Read the model definition and answer for the solid it produces. Units are mm, in the model's axes. Face numbers are marked on the shaded views. Give positions to 0.01 mm unless a question says otherwise; leave off trailing zeros. Write each loop counter-clockwise with the first axis right and the second up, starting at its lowest first coordinate (ties: lowest second). Pieces come first, ordered by that corner, then holes. Notation, with made-up numbers: (81.25, 55) -> (87.25, 55) arc R26 cw to (87.25, 78) -> close; hole circle Ø7 at (-24.5, 42.25). An arc over 180 degrees is marked (long way). Use a Markdown table: item, result.
from build123d import *

# Parameters (mm, degrees)
SKETCH_1_W                          = 1077
SKETCH_1_H                          = 1947
SM_BASE_FLANGE_1_DEPTH              = 2
SM_EDGE_FLANGE_1_STRIP_W            = 9.5
SM_EDGE_FLANGE_1_STRIP_H            = 2
SM_EDGE_FLANGE_1_STRIP_CUT_DEPTH    = 1947
SM_EDGE_FLANGE_1_STRIP_2_W          = 9.5
SM_EDGE_FLANGE_1_STRIP_2_H          = 2
SM_EDGE_FLANGE_1_STRIP_CUT_2_DEPTH  = 1947
SM_EDGE_FLANGE_1_DEPTH              = 1947
SM_EDGE_FLANGE_1_BEND_DEPTH         = 1947
SM_EDGE_FLANGE_2_STRIP_W            = 9.5
SM_EDGE_FLANGE_2_STRIP_H            = 2
SM_EDGE_FLANGE_2_STRIP_CUT_DEPTH    = 1031.5
SM_EDGE_FLANGE_2_RELIEF_W           = 10.5
SM_EDGE_FLANGE_2_RELIEF_H           = 1
SM_EDGE_FLANGE_2_RELIEF_CUT_DEPTH   = 2
SM_EDGE_FLANGE_2_STRIP_2_W          = 9.5
SM_EDGE_FLANGE_2_STRIP_2_H          = 2
SM_EDGE_FLANGE_2_STRIP_CUT_2_DEPTH  = 1031.5
SM_EDGE_FLANGE_2_RELIEF_2_W         = 10.5
SM_EDGE_FLANGE_2_RELIEF_2_H         = 1
SM_EDGE_FLANGE_2_RELIEF_CUT_2_DEPTH = 2
SM_EDGE_FLANGE_2_DEPTH              = 1031.5
SM_EDGE_FLANGE_2_BEND_DEPTH         = 1031.5


# Sheet-metal steps are written as plain solids
with BuildPart() as part:
    # Sketch 1 → Базовая кромка1 (new body)
    with BuildSketch(Plane.XY):
        Rectangle(SKETCH_1_W, SKETCH_1_H)
    extrude(amount=SM_BASE_FLANGE_1_DEPTH)

    # Ребро-кромка1 strip (across the edge) → Ребро-кромка1 strip cut (cut)
    with BuildSketch(Plane(origin=(-538.5, -973.5, 0), x_dir=(1, 0, 0), z_dir=(0, 1, 0))):
        with Locations((-2, -1)):
            Rectangle(SM_EDGE_FLANGE_1_STRIP_W, SM_EDGE_FLANGE_1_STRIP_H)
    extrude(amount=SM_EDGE_FLANGE_1_STRIP_CUT_DEPTH, mode=Mode.SUBTRACT)

    # Ребро-кромка1 strip 2 (across the edge) → Ребро-кромка1 strip cut 2 (cut)
    with BuildSketch(Plane(origin=(538.5, 973.5, 0), x_dir=(-1, 0, 0), z_dir=(0, -1, 0))):
        with Locations((-2, -1)):
            Rectangle(SM_EDGE_FLANGE_1_STRIP_2_W, SM_EDGE_FLANGE_1_STRIP_2_H)
    extrude(amount=SM_EDGE_FLANGE_1_STRIP_CUT_2_DEPTH, mode=Mode.SUBTRACT)

    # Ребро-кромка1 section (across the edge) → Ребро-кромка1 (add)
    with BuildSketch(Plane(origin=(-538.5, -973.5, 0), x_dir=(1, 0, 0), z_dir=(0, 1, 0))):
        with BuildLine():
            Line((0, 0.75), (0, 13))
            Line((0, 13), (2, 13))
            Line((2, 13), (2, 0.75))
            ThreePointArc((2, 0.75), (2.219669914, 0.219669914), (2.75, 0))
            Line((2.75, 0), (2.75, -2))
            ThreePointArc((2.75, -2), (0.805456352, -1.194543648), (0, 0.75))
        make_face()
    extrude(amount=SM_EDGE_FLANGE_1_DEPTH)

    # Ребро-кромка1 section 2 (across the edge) → Ребро-кромка1 bend (add)
    with BuildSketch(Plane(origin=(538.5, 973.5, 0), x_dir=(-1, 0, 0), z_dir=(0, -1, 0))):
        with BuildLine():
            Line((0, 0.75), (0, 13))
            Line((0, 13), (2, 13))
            Line((2, 13), (2, 0.75))
            ThreePointArc((2, 0.75), (2.219669914, 0.219669914), (2.75, 0))
            Line((2.75, 0), (2.75, -2))
            ThreePointArc((2.75, -2), (0.805456352, -1.194543648), (0, 0.75))
        make_face()
    extrude(amount=SM_EDGE_FLANGE_1_BEND_DEPTH)

    # Ребро-кромка2 strip (across the edge) → Ребро-кромка2 strip cut (cut)
    with BuildSketch(Plane(origin=(-515.75, 973.5, 0), x_dir=(0, -1, 0), z_dir=(1, 0, 0))):
        with Locations((-2, -1)):
            Rectangle(SM_EDGE_FLANGE_2_STRIP_W, SM_EDGE_FLANGE_2_STRIP_H)
    extrude(amount=SM_EDGE_FLANGE_2_STRIP_CUT_DEPTH, mode=Mode.SUBTRACT)

    # Ребро-кромка2 relief (on the sheet) → Ребро-кромка2 relief cut (cut)
    with BuildSketch(Plane(origin=(-515.75, 970.75, 0), x_dir=(0, -1, 0), z_dir=(0, 0, -1))):
        with Locations((-4.25, 0.5)):
            Rectangle(SM_EDGE_FLANGE_2_RELIEF_W, SM_EDGE_FLANGE_2_RELIEF_H)
        with Locations((-4.25, -1032)):
            Rectangle(SM_EDGE_FLANGE_2_RELIEF_W, SM_EDGE_FLANGE_2_RELIEF_H)
    extrude(amount=-SM_EDGE_FLANGE_2_RELIEF_CUT_DEPTH, mode=Mode.SUBTRACT)

    # Ребро-кромка2 strip 2 (across the edge) → Ребро-кромка2 strip cut 2 (cut)
    with BuildSketch(Plane(origin=(515.75, -973.5, 0), x_dir=(0, 1, 0), z_dir=(-1, 0, 0))):
        with Locations((-2, -1)):
            Rectangle(SM_EDGE_FLANGE_2_STRIP_2_W, SM_EDGE_FLANGE_2_STRIP_2_H)
    extrude(amount=SM_EDGE_FLANGE_2_STRIP_CUT_2_DEPTH, mode=Mode.SUBTRACT)

    # Ребро-кромка2 relief 2 (on the sheet) → Ребро-кромка2 relief cut 2 (cut)
    with BuildSketch(Plane(origin=(515.75, -970.75, 0), x_dir=(0, 1, 0), z_dir=(0, 0, -1))):
        with Locations((-4.25, 0.5)):
            Rectangle(SM_EDGE_FLANGE_2_RELIEF_2_W, SM_EDGE_FLANGE_2_RELIEF_2_H)
        with Locations((-4.25, -1032)):
            Rectangle(SM_EDGE_FLANGE_2_RELIEF_2_W, SM_EDGE_FLANGE_2_RELIEF_2_H)
    extrude(amount=-SM_EDGE_FLANGE_2_RELIEF_CUT_2_DEPTH, mode=Mode.SUBTRACT)

    # Ребро-кромка2 section (across the edge) → Ребро-кромка2 (add)
    with BuildSketch(Plane(origin=(-515.75, 973.5, 0), x_dir=(0, -1, 0), z_dir=(1, 0, 0))):
        with BuildLine():
            Line((0, 0.75), (0, 13))
            Line((0, 13), (2, 13))
            Line((2, 13), (2, 0.75))
            ThreePointArc((2, 0.75), (2.219669914, 0.219669914), (2.75, 0))
            Line((2.75, 0), (2.75, -2))
            ThreePointArc((2.75, -2), (0.805456352, -1.194543648), (0, 0.75))
        make_face()
    extrude(amount=SM_EDGE_FLANGE_2_DEPTH)

    # Ребро-кромка2 section 2 (across the edge) → Ребро-кромка2 bend (add)
    with BuildSketch(Plane(origin=(515.75, -973.5, 0), x_dir=(0, 1, 0), z_dir=(-1, 0, 0))):
        with BuildLine():
            Line((0, 0.75), (0, 13))
            Line((0, 13), (2, 13))
            Line((2, 13), (2, 0.75))
            ThreePointArc((2, 0.75), (2.219669914, 0.219669914), (2.75, 0))
            Line((2.75, 0), (2.75, -2))
            ThreePointArc((2.75, -2), (0.805456352, -1.194543648), (0, 0.75))
        make_face()
    extrude(amount=SM_EDGE_FLANGE_2_BEND_DEPTH)


solid = part.part
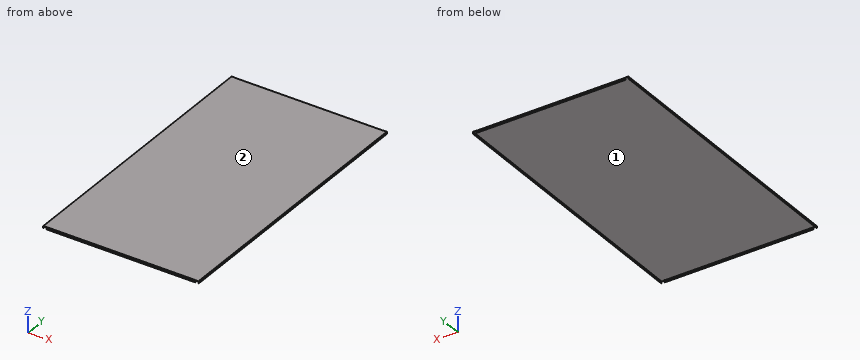
Item 1: A cutting plane is placed at C-C (y = -797). Give the vertices of the cut face in (x, z), then the cut area to 3 significant figures.
Return value:
| item | result |
|---|---|
| outline | (-538.5, -13) -> (-536.5, -13) -> (-536.5, -0.75) arc R0.75 cw to (-535.75, 0) -> (535.75, 0) arc R0.75 cw to (536.5, -0.75) -> (536.5, -13) -> (538.5, -13) -> (538.5, -0.75) arc R2.75 ccw to (535.75, 2) -> (-535.75, 2) arc R2.75 ccw to (-538.5, -0.75) -> close |
| area | 2,200 mm^2 |
Item 2: Straight lines are drawn through the part: line 1 along X through (y, z) = (-670, -2.5); line 2 along Y through (x, z) = (-349, -3.75); line 3 along Z through (x, y) = (-171.5, 374.5). For each, find the intervals that lie inside material, in ascending order. Write a range as [from, to].
Return value:
| item | result |
|---|---|
| line 1 | [-538.5, -536.5], [536.5, 538.5] |
| line 2 | [-973.5, -971.5], [971.5, 973.5] |
| line 3 | [0, 2] |
Item 3: A cutting plane is placed at B-B (x = -427.5). Give the vertices of the cut face in (y, z), then the cut area to 3 significant figures.
Return value:
| item | result |
|---|---|
| outline | (-973.5, -13) -> (-971.5, -13) -> (-971.5, -0.75) arc R0.75 cw to (-970.75, 0) -> (970.75, 0) arc R0.75 cw to (971.5, -0.75) -> (971.5, -13) -> (973.5, -13) -> (973.5, -0.75) arc R2.75 ccw to (970.75, 2) -> (-970.75, 2) arc R2.75 ccw to (-973.5, -0.75) -> close |
| area | 3,940 mm^2 |
Item 4: Each of these flat-tipped pins is pushed along its axis until it touches: P1, Ø8, axis at x = 263.5, y = -413.5, coming from the -Z side; P2, Ø0.6, axis at y = -972.5, z = 1.5, coming from the -X side; P3, Ø2, axis at y = 972, z = 1.5, coming from the -X side; P4, Ø3, axis at x = 42, z = 0, coming from the +Y side. Where does it stop, or does it pass through?
Return value:
| item | result |
|---|---|
| P1 | z = 0 |
| P2 | x = -537.69 |
| P3 | x = -538.2 |
| P4 | y = 973.5 |
Item 5: A cutting plane is placed at A-A (z = -3.25). Give the vertices of the cut face in (x, y), then the cut area to 3 significant figures.
Return value:
| item | result |
|---|---|
| outline | (-538.5, -973.5) -> (-536.5, -973.5) -> (-536.5, 973.5) -> (-538.5, 973.5) -> close; (-515.75, -973.5) -> (515.75, -973.5) -> (515.75, -971.5) -> (-515.75, -971.5) -> close; (-515.75, 971.5) -> (515.75, 971.5) -> (515.75, 973.5) -> (-515.75, 973.5) -> close; (536.5, -973.5) -> (538.5, -973.5) -> (538.5, 973.5) -> (536.5, 973.5) -> close |
| area | 11,900 mm^2 |
Item 6: For a pull along Y with two mould halves and no side action, classify the marked faces 1 and 2 as +Y half, -Y half, draft (parallel to the pull), parting line (faces both ways), or undercut.
Return value:
| item | result |
|---|---|
| face 1 | undercut |
| face 2 | draft |
